from build123d import *

# Parameters (mm, degrees)
SKETCH1_R           = 7.5
BOSS_EXTRUDE1_DEPTH = 45
SKETCH2_W           = 5
SKETCH2_H           = 4.459975541
CUT_EXTRUDE1_DEPTH  = 30


with BuildPart() as part:
    # Sketch1 → Boss-Extrude1 (new body)
    with BuildSketch(Plane.XY):
        Circle(SKETCH1_R)
    extrude(amount=BOSS_EXTRUDE1_DEPTH)

    # Sketch2 → Cut-Extrude1 (cut)
    with BuildSketch(Plane.XY.offset(45)):
        with Locations((0, 7.229987771)):
            Rectangle(SKETCH2_W, SKETCH2_H)
    extrude(amount=-CUT_EXTRUDE1_DEPTH, mode=Mode.SUBTRACT)


solid = part.part
Input: part model. Units: mm. Frame: model coordinates. A direction names the side the tool comes from. Give positions to 0.01 mm unless a question says otherwise; leave off trailing zeros. Write each loop counter-clockwise with the first axis right and the second up, starting at its lowest first coordinate (ties: lowest second). Pieces come first, ordered by that corner, then holes. Notation, with made-up numbers: M -29.5,58.5 L 17.5,58.5 A23 cw 17.5,97.5 Z; hole C -30.5,61 d6. An arc over 180 degrees is marked long. Write item = value, one per line. Start each with the question number.
1) Draft query along X for faces 1 (the flat face through (2.5, 6, 30)), 2 (the flat face through (0, 0, 45)), 3 (the cylindrical face through (-1.63, -7.32, 22.18)). Return one class per face: +X half, -X half, draft (parallel to the pull), parting line (faces both ways), or undercut.
2) Reachability of faces 4 (the flat face through (-2.5, 6, 30)), 5 (the flat face through (0, 0, 0)) from +Z, -Z, +X, -X, +Y, -Y: full face, straight path, thin tool, end or side. Return the list, or none.
3) Cut plane A-A on x = 0. Return the cut outline in (y, z), then the cut area to 3 significant figures.
4) Cut plane B-B on z = 11.5. Return the cut outline in (x, y), then the cut area to 3 significant figures.
5) Cut plane C-C on y = -6.5. Return the cut outline in (x, z).
6) Material intervals for line 1 along Y through (x, z) = (0.25, 41.5); line 2 along Z through (x, y) = (1.25, 6.25); line 3 along X through (y, z) = (-1.75, 34), sorted ascending. Write a range as [from, to].
7) First-contact query: pin 1 Ø5.5 at (x, z) = (-1, 28) entering from +Y; pin 2 Ø1 at (x, z) = (-3.5, 27) entering from +Y; pin 3 Ø4 at (y, z) = (5, 23.5) entering from +X. Flat tips, straight axial feed; report the tip coordinate or a pass-through.
8) Cut plane D-D on z = 17.5. Return the cut outline in (x, y).
Solved:
q1.face_1 = undercut
q1.face_2 = draft
q1.face_3 = parting line
q2.face_4 = +Z, +Y
q2.face_5 = -Z, +X, -X, +Y, -Y
q3.outline = M -7.5,0 L 7.5,0 L 7.5,15 L 5,15 L 5,45 L -7.5,45 Z
q3.area = 600 mm2
q4.outline = C 0,0 d15
q4.area = 177 mm2
q5.outline = M -3.74,0 L 3.74,0 L 3.74,45 L -3.74,45 Z
q6.line_1 = [-7.5, 5]
q6.line_2 = [0, 15]
q6.line_3 = [-7.29, 7.29]
q7.pin_1 = 7.07
q7.pin_2 = 6.87
q7.pin_3 = 6.87
q8.outline = M -2.5,5 L -2.5,7.07 A7.5 ccw long 2.5,7.07 L 2.5,5 Z
